Input: dimensioned drawing with shaded views. Units: mm. Origin: part minimum x, y, z. A direction names the side the tool comes from. Coordinates: 2 decimals unless noted, no trailing zeros. Loops run counter-clockwise (first coordinate to the right, second up) from the corner with the lowest first, then second, coordinate; pieces in that order, holes last.
Item 1: Line query: probe 1 along Y at (x, z) = (2.5, 10); probe 2 along Z at (x, y) = (1.8, 10); probe 3 along Z at (x, y) = (1.5, 5.25). Output: solid intervals per line, ascending.
Item 2: Reachability of the marked faces 5, 6 and 7 from +Z, -Z, +X, -X, +Y, -Y: full face, straight path, thin tool, end or side. Return the list, or none.
Item 3: Section query D-D, the plane z = 18.75. Return the cut outline in (x, y).
Item 4: Pin query (flat end, axial travel): pin 1 Ø1.5 at (x, y) = (3.5, 8) entering from -Z; pin 2 Ø1.5 at (x, y) = (1.5, 14) entering from +Z. Return the tip coordinate at first contact, or that it passes through.
Item 5: Section query C-C, the plane y = 4. Return the cut outline in (x, z).
Item 6: Section query A-A, the plane x = 4.6. Return the cut outline in (y, z).
Item 7: Section query B-B, the plane z = 10. Return the cut outline in (x, y).
Item 8: Pull-direction query (Z, two-part tool) for the marked faces 1, 2, 3 and 4; classes: +Z half, -Z half, draft (parallel to the pull), parting line (faces both ways), or undercut.
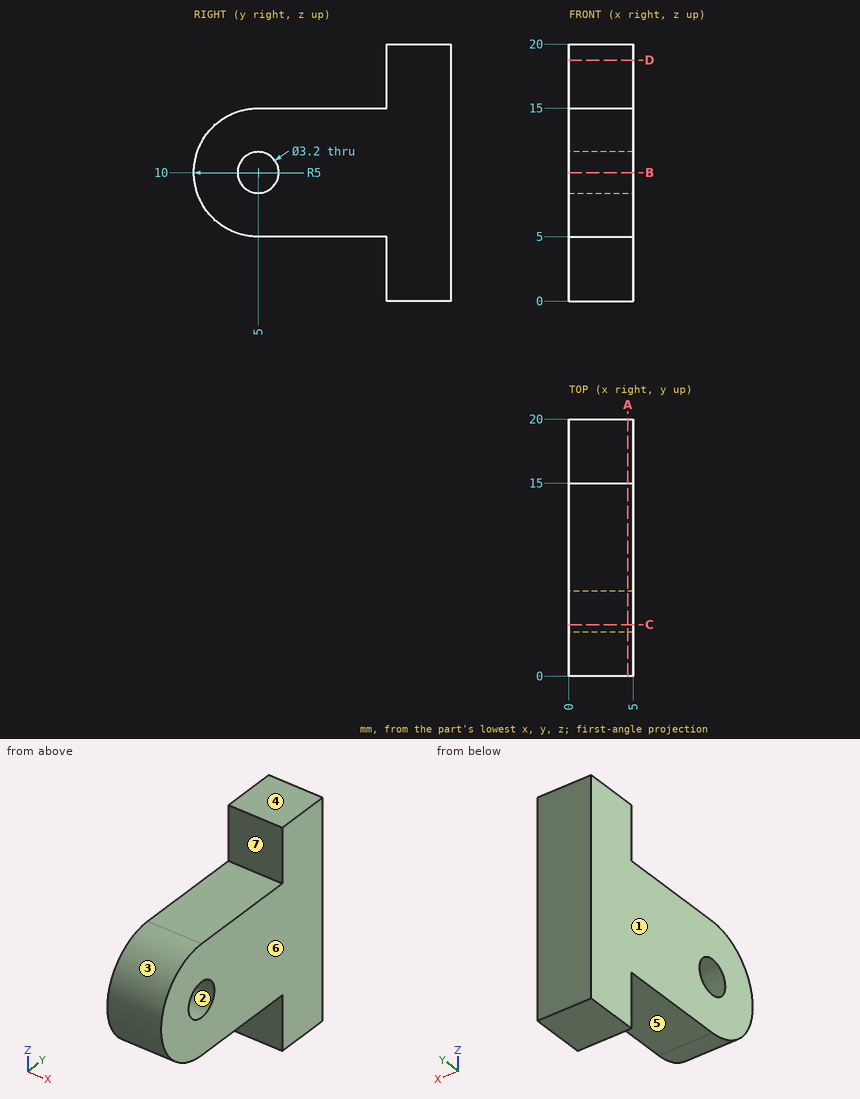
Verdict:
1. probe 1: y = 0 to 3.4, 6.6 to 20
1. probe 2: z = 5 to 15
1. probe 3: z = 5 to 8.42, 11.58 to 15
2. face 5: -Z, +X, -X, -Y
2. face 6: +Z, -Z, +X, +Y, -Y
2. face 7: +Z, +X, -X, -Y
3. outline: (0, 15) - (5, 15) - (5, 20) - (0, 20) - close
4. pin 1: stops at z = 5
4. pin 2: stops at z = 15
5. outline: (0, 5.1) - (5, 5.1) - (5, 8.75) - (0, 8.75) - close; (0, 11.25) - (5, 11.25) - (5, 14.9) - (0, 14.9) - close
6. outline: (5, 5) - (15, 5) - (15, 0) - (20, 0) - (20, 20) - (15, 20) - (15, 15) - (5, 15) arc R5 ccw to start; hole circle Ø3.2 at (5, 10)
7. outline: (0, 0) - (5, 0) - (5, 3.4) - (0, 3.4) - close; (0, 6.6) - (5, 6.6) - (5, 20) - (0, 20) - close
8. face 1: draft
8. face 2: undercut
8. face 3: parting line
8. face 4: +Z half
